from build123d import *

# Parameters (mm, degrees)
EXTRUDE1_DEPTH     = 150
CUT_EXTRUDE1_REACH = 78
SKETCH2_R          = 8.5


with BuildPart() as part:
    # Sketch1 → Extrude1 (new body, symmetric)
    with BuildSketch(Plane(origin=(0, 0, 0), x_dir=(1, 0, 0), z_dir=(0, 1, 0))):
        with BuildLine():
            Line((-127, 0), (127, 0))
            Line((127, 0), (127, 76))
            ThreePointArc((127, 76), (121.343145751, 73.656854249), (119, 68))
            Line((119, 68), (119, 14))
            ThreePointArc((119, 14), (117.242640687, 9.757359313), (113, 8))
            Line((113, 8), (-113, 8))
            ThreePointArc((-113, 8), (-117.242640687, 9.757359313), (-119, 14))
            Line((-119, 14), (-119, 68))
            ThreePointArc((-119, 68), (-121.343145751, 73.656854249), (-127, 76))
            Line((-127, 76), (-127, 0))
        make_face()
    extrude(amount=EXTRUDE1_DEPTH, both=True)

    # Sketch2 → Cut-Extrude1 (cut, up to next)
    with BuildSketch(Plane.XY, mode=Mode.PRIVATE) as cut_extrude1_sk1:
        with Locations((84, 70)):
            Circle(SKETCH2_R)
    cut_extrude1_tool1 = extrude(cut_extrude1_sk1.sketch, amount=-CUT_EXTRUDE1_REACH, mode=Mode.PRIVATE) & part.part
    add(cut_extrude1_tool1.solids().sort_by_distance((84, 70, 0))[0], mode=Mode.SUBTRACT)
    # Sketch2 → Cut-Extrude1 (cut, up to next)
    with BuildSketch(Plane.XY, mode=Mode.PRIVATE) as cut_extrude1_sk2:
        with Locations((-84, 70)):
            Circle(SKETCH2_R)
    cut_extrude1_tool2 = extrude(cut_extrude1_sk2.sketch, amount=-CUT_EXTRUDE1_REACH, mode=Mode.PRIVATE) & part.part
    add(cut_extrude1_tool2.solids().sort_by_distance((-84, 70, 0))[0], mode=Mode.SUBTRACT)
    # Sketch2 → Cut-Extrude1 (cut, up to next)
    with BuildSketch(Plane.XY, mode=Mode.PRIVATE) as cut_extrude1_sk3:
        with Locations((-84, -70)):
            Circle(SKETCH2_R)
    cut_extrude1_tool3 = extrude(cut_extrude1_sk3.sketch, amount=-CUT_EXTRUDE1_REACH, mode=Mode.PRIVATE) & part.part
    add(cut_extrude1_tool3.solids().sort_by_distance((-84, -70, 0))[0], mode=Mode.SUBTRACT)
    # Sketch2 → Cut-Extrude1 (cut, up to next)
    with BuildSketch(Plane.XY, mode=Mode.PRIVATE) as cut_extrude1_sk4:
        with Locations((84, -70)):
            Circle(SKETCH2_R)
    cut_extrude1_tool4 = extrude(cut_extrude1_sk4.sketch, amount=-CUT_EXTRUDE1_REACH, mode=Mode.PRIVATE) & part.part
    add(cut_extrude1_tool4.solids().sort_by_distance((84, -70, 0))[0], mode=Mode.SUBTRACT)


solid = part.part
Here's how the part is built. I have some questions about the finished solid (model axes, mm). A direction names the side the tool comes from. Coordinates: 2 decimals unless noted, no trailing zeros. Order: outer loops, then holes, each group sorted by start corner. A loop starts at its lowest first (then second) coordinate and runs counter-clockwise, first axis right, second up. Notation, with made-up numbers: (31, 20.5) - (90, 20.5) arc R20 cw to (90, 30.5) - close; hole circle Ø7 at (-1.75, 10.5). An arc over 180 degrees is marked (long way). Use CSV: the item, a comma, the result in double quotes. Start each with the question number.
1. For faces 1 (the face through (-119, 2, -41)), 2 (the face through (-92.49, -69.63, -3.94)), which set-ups out of +Z, -Z, +X, -X, +Y, -Y let a thin tool reach every point of the face, with its end or its side?
2. Suppose I cut it at C-C on z = -19. List the corners of the cut face in (x, y) for me, then the cut area to 3 significant figures.
3. Please list where these lines run through material, in increasing order: line 1 (Y direction, x = -84, z = -3.75); line 2 (X direction, y = -29, z = -27); line 3 (X direction, y = -128, z = -69). Write a range as from..to.
4. If we mould it in two halves opening along X, with no side actions, what happens to faces 3 (the face through (127, 2, -37)), 4 (the face through (2, 2, -8)), 5 (the face through (-1, -150, -7))? For each: +X half, -X half, draft (parallel to the pull), parting line (faces both ways), or undercut.
5. I'm going to push flat-ended pins straight in: pin 1 (13.5 mm diameter, centred on x = 84, y = 70, fed in from +Z); pin 2 (5 mm diameter, centred on x = -20, y = 87.5, fed in from -Z). Where does each tip first touch, or does it pass through?
6. Suppose I cut it at B-B on x = -84. List the corners of the cut face in (y, z) for me.
7. Suppose I cut it at A-A on y = 70. List the corners of the cut face in (x, z) for me.
Output:
1,face 1,"-Z, +Y, -Y"
1,face 2,"+Z, -Z"
2,outline,"(-127, -150) - (-119, -150) - (-119, 150) - (-127, 150) - close; (119, -150) - (127, -150) - (127, 150) - (119, 150) - close"
2,area,"4,800 mm2"
3,line 1,"y = -150..-78.5, -61.5..61.5, 78.5..150"
3,line 2,"x = -127..-119, 119..127"
3,line 3,"x = -127..-119.06, 119.06..127"
4,face 3,"+X half"
4,face 4,"undercut"
4,face 5,"draft"
5,pin 1,"passes through"
5,pin 2,"stops at z = -8"
6,outline,"(-150, -8) - (-78.5, -8) - (-78.5, 0) - (-150, 0) - close; (-61.5, -8) - (61.5, -8) - (61.5, 0) - (-61.5, 0) - close; (78.5, -8) - (150, -8) - (150, 0) - (78.5, 0) - close"
7,outline,"(-127, -76) arc R8 ccw to (-119, -68) - (-119, -14) arc R6 cw to (-113, -8) - (-92.5, -8) - (-92.5, 0) - (-127, 0) - close; (-75.5, -8) - (75.5, -8) - (75.5, 0) - (-75.5, 0) - close; (92.5, -8) - (113, -8) arc R6 cw to (119, -14) - (119, -68) arc R8 ccw to (127, -76) - (127, 0) - (92.5, 0) - close"
